Build history of the part. All positions in model axes, mm. A direction names the side the tool comes from. Give positions to 0.01 mm unless a question says otherwise; leave off trailing zeros. Loops run counter-clockwise (first coordinate to the right, second up) from the corner with the lowest first, then second, coordinate; pieces in that order, holes last. Notation, with made-up numbers: M 37,51.5 L 81,51.5 A16 ccw 81,79.5 Z; hole C -9.5,23 d9. An arc over 180 degrees is marked long. Answer as a JSON object with one key per item and string values. Group by question number.
1. Slice it at A-A (x = 0). List the corners of the cut face in (y, z).
2. Drop flat-ended pins along their axis: pin 1 Ø2 at (x, y) = (-0.5, -2) entering from +Z; pin 2 Ø2 at (x, z) = (-1.5, -5) entering from +Y; pin 3 Ø2 at (x, z) = (0.5, -11.5) entering from -Y; pin 4 Ø12 at (y, z) = (-7, -10) entering from +X. Give the stop position or say it passes through.
3. Slice it at B-B (z = -15). List the corners of the cut face in (x, y).
4. Slice it at C-C (y = 3.5). List the corners of the cut face in (x, z).
5. Drill centre lines: line 1 along Y through (x, z) = (-1.35, -15); line 2 along X through (y, z) = (-0.5, 1); line 3 along Z through (x, y) = (0.5, -1). Where is each one in solid material? Low to high. Write a range as [from, to].
6. 3-axis set-ups, long thin cutter, end or side, ignore diameter. For faces 1 (the face through (-1.755, -14.309, -17.008)), 2 (the face through (0, -13, -21.438)), 3 (the face through (-1.89, 6.26, -1.45)): which of +Z, -Z, +X, -X, +Y, -Y reach the whole face in a straight line?
7. Slice it at D-D (x = 1.6). List the corners of the cut face in (y, z), then the cut area to 3 significant figures.
from build123d import *

# Parameters (mm, degrees)
F0_R     = 2.38125
F1_ANGLE = 90
F2_DEPTH = 8.7376
F3_DEPTH = 12.7


with BuildPart() as f1:
    # F0 (on Front) → F1 (revolve)
    with BuildSketch(Plane.XZ):
        Circle(F0_R)
    revolve(axis=Axis((1.0816315189, 0, -12.7), (1, 0, 0)), revolution_arc=F1_ANGLE)

    # F2 (add): a face of the model
    f2_faces = [f1.faces().sort_by_distance(p)[0] for p in [
        (0, -12.7, -12.7),
    ]]
    extrude(f2_faces, amount=F2_DEPTH)

    # F3 (add): a face of the model
    f3_faces = [f1.faces().sort_by_distance(p)[0] for p in [
        (0, 0, 0),
    ]]
    extrude(f3_faces, amount=F3_DEPTH)


solid = f1.part
Established:
{
 "1": {"outline": "M -15.08,-21.44 L -10.32,-21.44 L -10.32,-12.7 A10.32 cw 0,-2.38 L 12.7,-2.38 L 12.7,2.38 L 0,2.38 A15.08 ccw -15.08,-12.7 Z"},
 "2": {"pin 1": "stops at z = 2.34", "pin 2": "stops at y = -6.14", "pin 3": "stops at y = -15.08", "pin 4": "stops at x = 2.38"},
 "3": {"outline": "C 0,-12.7 d4.76"},
 "4": {"outline": "C 0,0 d4.76"},
 "5": {"line 1": "y = [-14.66, -10.74]", "line 2": "x = [-2.16, 2.16]", "line 3": "z = [-2.38, 2.29]"},
 "6": {"face 1": "-Z", "face 2": "-Z, +X, -X, +Y, -Y", "face 3": "+Y"},
 "7": {"outline": "M -14.46,-21.44 L -10.94,-21.44 L -10.94,-12.7 A10.94 cw 0,-1.76 L 12.7,-1.76 L 12.7,1.76 L 0,1.76 A14.46 ccw -14.46,-12.7 Z", "area": "146 mm^2"}
}
